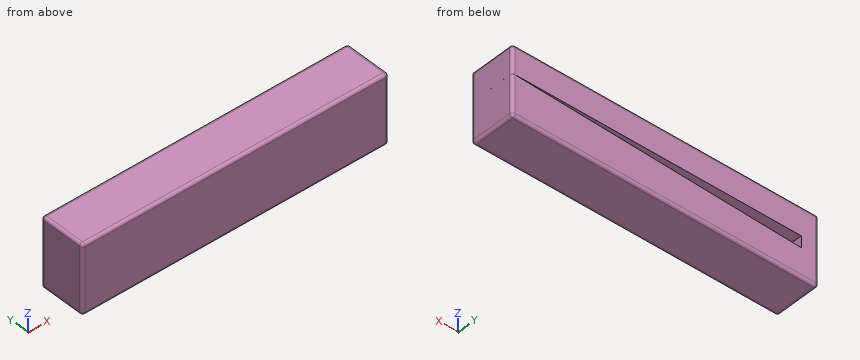
from build123d import *

# Parameters (mm, degrees)
SKETCH1_W             = 50
SKETCH1_H             = 5
BOSS_EXTRUDE1_DEPTH   = 5
BOSS_EXTRUDE1_2_DEPTH = 5
SKETCH2_W             = 50
SKETCH2_H             = 12
BOSS_EXTRUDE2_DEPTH   = 3
SKETCH3_W             = 3
SKETCH3_H             = 12
BOSS_EXTRUDE3_DEPTH   = 8
FILLET1_R             = 0.5


with BuildPart() as part:
    # Sketch1 → Boss-Extrude1 (new body)
    with BuildSketch(Plane(origin=(0, 0, 0), x_dir=(1, 0, 0), z_dir=(0, 1, 0))):
        with Locations((25, -3.5)):
            Rectangle(SKETCH1_W, SKETCH1_H)
    extrude(amount=BOSS_EXTRUDE1_DEPTH)



with BuildPart() as body_2:
    # Sketch1 → Boss-Extrude1 2 (new body)
    with BuildSketch(Plane(origin=(0, 0, 0), x_dir=(1, 0, 0), z_dir=(0, 1, 0))):
        Polygon((0, 6), (0, 1), (50, -0.998001998), (50, 6), align=None)
    extrude(amount=BOSS_EXTRUDE1_2_DEPTH)


with BuildPart() as body_3:
    # Sketch2 → Boss-Extrude2 (new body)
    with BuildSketch(Plane.XZ):
        with Locations((25, 0)):
            Rectangle(SKETCH2_W, SKETCH2_H)
    extrude(amount=BOSS_EXTRUDE2_DEPTH)


with BuildPart() as part_1:
    add(part.part)

    add(body_2.part)  # Boss-Extrude3 merges body 2

    add(body_3.part)  # Boss-Extrude3 merges body 3
    # Sketch3 → Boss-Extrude3 (add)
    with BuildSketch(Plane.XZ.offset(3)):
        with Locations((-1.5, 0)):
            Rectangle(SKETCH3_W, SKETCH3_H)
    extrude(amount=-BOSS_EXTRUDE3_DEPTH)

    # Fillet1
    fillet1_edges = [part_1.edges().sort_by_distance(p)[0] for p in [
        (23.5, 5, -6),
        (-3, 5, 0),
        (-3, 1, -6),
        (-3, 1, 6),
        (23.5, -3, 6),
        (-3, -3, 0),
        (23.5, -3, -6),
        (23.5, 5, 6),
        (50, 5, -2.500999001),
        (50, 1, -6),
        (50, -3, 0),
        (50, 5, 3.5),
        (50, 1, 6),
    ]]
    fillet(fillet1_edges, radius=FILLET1_R)


solid = part_1.part
Verification items for the finished model (mm, model axes). Round coordinates to 2 decimals unless told otherwise and drop trailing zeros. Loops run counter-clockwise (first coordinate to the right, second up) from the corner with the lowest first, then second, coordinate; pieces in that order, holes last. Notation, with made-up numbers: (65, -13.5) - (89, -13.5) arc R22 ccw to (89, -4.5) - close; hole circle Ø4 at (28.25, -6). An arc over 180 degrees is marked (long way). Use a Markdown table: item, result. Add a question column.
1. Section check B-B, the plane y = 2.75. Record the boundary of the cut face in (x, z), plus the area to 3 significant figures.
2. Thickness scan on probe 1 along Y at (x, z) = (10, -0.25); probe 2 along Z at (x, y) = (3, 2.75); probe 3 along Z at (x, y) = (39.5, 3.75). Record the ranges inside material, lowest first. Write a range as [from, to].
3. Gauge pin test, flat end, axial feed: pin 1 (2 mm diameter, centred on x = 19, z = 0, fed in from +Y). Record the tip position at first contact, or that the pin passes through.
4. Section check A-A, the plane z = 0. Record the boundary of the cut face in (x, y) (3 decimals).
Checks:
| question | item | result |
|---|---|---|
| 1 | outline | (-3, -5.5) arc R0.5 ccw to (-2.5, -6) - (49.5, -6) arc R0.5 ccw to (50, -5.5) - (50, 1) - (0, -1) - (0, 1) - (50, 1) - (50, 5.5) arc R0.5 ccw to (49.5, 6) - (-2.5, 6) arc R0.5 ccw to (-3, 5.5) - close |
| 1 | area | 586 mm^2 |
| 2 | probe 1 | y = [-3, 0] |
| 2 | probe 2 | z = [-6, -0.88], [1, 6] |
| 2 | probe 3 | z = [-6, 0.58], [1, 6] |
| 3 | pin 1 | stops at y = 5 |
| 4 | outline | (-3, -2.5) arc R0.5 ccw to (-2.5, -3) - (49.5, -3) arc R0.5 ccw to (50, -2.5) - (50, 4.5) arc R0.5 ccw to (49.5, 5) - (25.025, 5) - (25.025, 0) - (0, 0) - (0, 5) - (-2.5, 5) arc R0.5 ccw to (-3, 4.5) - close |
